Design review of the part built by this model. Coordinates are the model's own, in mm. A direction names the side the tool comes from. Coordinates: 2 decimals unless noted, no trailing zeros. Write each loop counter-clockwise with the first axis right and the second up, starting at its lowest first coordinate (ties: lowest second). Pieces come first, ordered by that corner, then holes.
Q1. Take a section at D-D, the plane z = -3.5. Write out the cut boundary in (x, y), plus the area to 3 significant figures.
Q2. The part is to be moulded in two halves that separate along Y. For faces 1 (the flat face through (-0.2, 4, -0.2)), 2 (the cylindrical face through (23.46, -3.56, 0.35)), 3 (the flat face through (1, -8, -7)), 4 (the flat face through (-13, 2, -1)), say which applies: released by +Y, released by -Y, zero draft, split by the parting line, or undercut.
Q3. Take a section at A-A, the plane y = 2.25. Write out the cut boundary in (x, z).
Q4. For faces 5 (the flat face through (-10, 2, 0)), 6 (the flat face through (25, -2, -3)), 7 (the flat face through (-4, -4, 0)), list the 3-axis set-ups (+Z, -Z, +X, -X, +Y, -Y) from which the entire face can be reached by the end or side of a thin tool; tool diameter is ignored.
Q5. For pin 1 Ø1.9 at (y, z) = (-2, 0) entering from -X; pin 2 Ø5.5 at (x, z) = (-11.75, -8) entering from -Y, all flat-tipped, find the tip position at first contact; note any pin that passes through.
Q6. Take a section at B-B, the plane z = 0. Write out the cut boundary in (x, y).
Q7. For L1, parallel to Z at x = 11, y = 0.25; L2, parallel to X at y = 1.25, z = 8; L3, parallel to Y at x = 23, z = 0, list the stretches that pass through material, from the lowest coordinate up.
Q8. Take a section at C-C, the plane x = -11.75. Write out the cut boundary in (y, z).
Autodesk Inventor part; units mm, degrees
ref_plane "YZ Plane" through (0, 0, 0) normal (1, 0, 0) x (0, 1, 0)
ref_plane "XZ Plane" through (0, 0, 0) normal (0, 1, 0) x (-1, 0, 0)
ref_plane "XY Plane" through (0, 0, 0) normal (0, 0, 1) x (1, 0, 0)
sketch "Эскиз1" plane through (0, 0, 0) normal (0, 1, 0) x (-1, 0, 0)
  line L0 (0, 15) -> (10, 15)
  line L1 (10, 15) -> (10, -15)
  line L2 (10, -15) -> (0, -15)
  line L3 (0, -15) -> (0, 15)
  circle A0 centre (11.75, 8) radius 1.75
  circle A1 centre (11.75, -8) radius 1.75
  line L4 (15.75, 15) -> (7.75, 15)
  line L5 (7.75, 15) -> (7.75, 1)
  line L6 (7.75, 1) -> (15.75, 1)
  line L7 (15.75, 1) -> (15.75, 15)
  line L8 (15.75, 15) -> (7.75, 1) construction
  line L9 (7.75, 15) -> (15.75, 1) construction
  line L10 (15.75, -1) -> (7.75, -1)
  line L11 (7.75, -1) -> (7.75, -15)
  line L12 (7.75, -15) -> (15.75, -15)
  line L13 (15.75, -15) -> (15.75, -1)
  line L14 (15.75, -1) -> (7.75, -15) construction
  line L15 (7.75, -1) -> (15.75, -15) construction
  point P0 (0, 0)
  point P1 (10, -1)
  point P2 (10, 1)
  point P3 (10, 15)
  point P4 (0, 0)
  dimension "d0" = 10
  dimension "d1" = 30
  dimension "d2" = 3.5
  dimension "d3" = 3.5
  dimension "d4" = 7
  dimension "d5" = 7
  dimension "d6" = 4
  dimension "d7" = 4
extrude "Выдавливание1" add sketch "Эскиз1" along normal blind 4
sketch "Эскиз2" plane through (0, 0, 0) normal (0, -1, 0) x (1, 0, 0)
  line L0 (-15.75, 15) -> (0, 15)
  line L1 (0, -15) -> (-15.75, -15)
  line L2 (0, 15) -> (-4, 15)
  line L3 (-4, 15) -> (-4, -15)
  line L4 (-4, -15) -> (0, -15)
  line L5 (0, -15) -> (0, 15)
  line L6 (-10, -1) -> (-10, 1)
  line L7 (-10, 1) -> (-10, 15) construction
  line L8 (-15.75, 15) -> (0, 15)
  point P0 (0, 0)
  point P1 (-4, 15)
  point P2 (-10, 0)
  dimension "d27" = 6
extrude "Выдавливание2" add sketch "Эскиз2" along normal blind 8
sketch "Эскиз3" plane through (0, 4, 0) normal (0, 1, 0) x (1, 0, 0)
  circle A0 centre (11, 0) radius 11
  line L0 (-15.75, -15) -> (0, -15)
  line L1 (0, -15) -> (25, -15)
  line L2 (0, -15) -> (0, 15)
  line L3 (0, 15) -> (-15.75, 15)
  line L4 (0, 15) -> (25, 15)
  line L5 (25, 15) -> (25, -15)
  point P0 (0, 0)
  dimension "d13" = 22
  dimension "d14" = 11
  dimension "d15" = 14
extrude "Выдавливание3" add sketch "Эскиз3" against normal up to surface (12 mm away)
sketch "Эскиз4" plane through (25, 4, 15) normal (1, 0, 0) x (0, 0, -1)
  line L0 (0, 0) -> (0, -12) construction
  line L1 (30, 0) -> (30, -12) construction
  line L2 (30, -4) -> (30, 0) construction
  line L3 (30, 0) -> (0, -12) construction
  circle A0 centre (15, -6) radius 1.6
  dimension "d19" = 3.2
extrude "Выдавливание4" cut sketch "Эскиз4" against normal blind 10
chamfer "Фаска1" distance 4 angle 45 2 edges at (25, -2, 15) (25, -2, -15)
properties part number "креп_маркера" material "Полипропилен"
Responses:
1. outline: (-15.75, 0) - (-4, 0) - (-4, -8) - (0.57, -8) - (0.57, 4) - (-15.75, 4) - close; (21.43, -8) - (25, -8) - (25, 4) - (21.43, 4) - close
1. area: 145 mm2
2. face 1: released by +Y
2. face 2: undercut
2. face 3: released by -Y
2. face 4: zero draft
3. outline: (-15.75, -15) - (21, -15) - (25, -11) - (25, 11) - (21, 15) - (-15.75, 15) - (-15.75, 1) - (-10, 1) - (-10, -1) - (-15.75, -1) - close; hole circle Ø3.5 at (-11.75, -8); hole circle Ø3.5 at (-11.75, 8); hole circle Ø22 at (11, 0)
4. face 5: -X, +Y, -Y
4. face 6: +Z, -Z, +X, +Y, -Y
4. face 7: +Z, -Z, -X, -Y
5. pin 1: stops at x = -4
5. pin 2: stops at y = 0
6. outline: (-10, 0) - (-4, 0) - (-4, -8) - (0, -8) - (0, 4) - (-10, 4) - close; (22, -8) - (25, -8) - (25, -3.6) - (22, -3.6) - close; (22, -0.4) - (25, -0.4) - (25, 4) - (22, 4) - close
7. L1: z = -15 to -11, 11 to 15
7. L2: x = -15.75 to -13.5, -10 to 3.45, 18.55 to 25
7. L3: y = -8 to -3.6, -0.4 to 4
8. outline: (0, -15) - (4, -15) - (4, -9.75) - (0, -9.75) - close; (0, -6.25) - (4, -6.25) - (4, -1) - (0, -1) - close; (0, 1) - (4, 1) - (4, 6.25) - (0, 6.25) - close; (0, 9.75) - (4, 9.75) - (4, 15) - (0, 15) - close
